from build123d import *

# Parameters (mm, degrees)
EXTRUDE_2_DEPTH      = 5
EXTRUDE_3_DEPTH      = 23.5
SKETCH_3_R           = 1.65
CUT_EXTRUDE_1_DEPTH  = 85.951456727
CUT_EXTRUDE_5_REACH  = 89.951
CUT_EXTRUDE_START    = 3
SKETCH_8_R           = 3
CUT_EXTRUDE_10_REACH = 89.951
CUT_EXTRUDE_START_2  = -3
SKETCH_12_R          = 3
SKETCH_4_W           = 20
SKETCH_4_H           = 10
CUT_EXTRUDE_2_DEPTH  = 5
SKETCH_10_W          = 16
SKETCH_10_H          = 40
CUT_EXTRUDE_11_DEPTH = 85.951456727
FILLET_1_R           = 3
CUT_EXTRUDE_6_DEPTH  = 94.465851734
SKETCH_6_R           = 2.6
CUT_EXTRUDE_3_DEPTH  = 83.421182124
CUT_EXTRUDE_4_REACH  = 89.421
CUT_EXTRUDE_START_3  = -5
SKETCH_7_R           = 4.4
FILLET_3_R           = 2
CUT_EXTRUDE_13_DEPTH = 90.709896


with BuildPart() as part:
    # 草图2 → 凸台-拉伸2 (new body)
    with BuildSketch(Plane(origin=(0, 0, 0), x_dir=(1, 0, 0), z_dir=(0, 1, 0))):
        Polygon((0, 0), (23.5, 0), (23.5, -19), (23.5, -80), (0, -80), align=None)
    extrude_2 = extrude(amount=EXTRUDE_2_DEPTH)

    # 镜向1: 凸台-拉伸2 across plane
    add(extrude_2.mirror(Plane(origin=(0, 5, 80), x_dir=(0, 0, 1), z_dir=(1, 0, 0))))

    # 草图5 → 凸台-拉伸3 (add, symmetric)
    with BuildSketch(Plane(origin=(0, 0, 0), x_dir=(0, 0, -1), z_dir=(1, 0, 0))):
        Polygon((-80, 0), (-16.263455967, -11.263455967), (-11.242997821, -6.242997821), (-9.192388155, -4.192388155), (-13.384776311, 0), align=None)
        Polygon((-13.384776311, 0), (-9.192388155, -4.192388155), (-7.14177849, -2.14177849), (-5, 0), align=None)
        Polygon((-7.14177849, -2.14177849), (-9.192388155, -4.192388155), (-8.838834765, -4.545941546), (-6.788225099, -2.495331881), align=None)
        Polygon((-9.192388155, -4.192388155), (-11.242997821, -6.242997821), (-10.88944443, -6.596551211), (-8.838834765, -4.545941546), align=None)
    extrude(amount=EXTRUDE_3_DEPTH, both=True)

    # 草图3 → 切除-拉伸1 (cut, through all)
    with BuildSketch(Plane(origin=(0, 5, 0), x_dir=(1, 0, 0), z_dir=(0, 1, 0))):
        with Locations(Location((-20, -20, 0), (0, 0, 270))):
            Circle(SKETCH_3_R)
        with Locations(Location((20, -20, 0), (0, 0, 270))):
            Circle(SKETCH_3_R)
        with Locations(Location((-20, -75, 0), (0, 0, 270))):
            Circle(SKETCH_3_R)
        with Locations(Location((20, -75, 0), (0, 0, 270))):
            Circle(SKETCH_3_R)
    extrude(amount=-CUT_EXTRUDE_1_DEPTH, mode=Mode.SUBTRACT)

    # 切除-拉伸5: up to this plane
    cut_extrude_5_end = Plane(origin=(23.5, -13.709378738, 2.422707194), z_dir=(0, 0.9847416717466503, -0.174022527063632))
    # 草图8 → 切除-拉伸5 (cut, up to the surface)
    with BuildSketch(Plane.XZ.offset(-5).offset(CUT_EXTRUDE_START), mode=Mode.PRIVATE) as cut_extrude_5_sk1:
        with Locations(Location((-20, 20, 0), (0, 0, 90))):
            Circle(SKETCH_8_R)
    cut_extrude_5_tool1 = split(extrude(cut_extrude_5_sk1.sketch, amount=CUT_EXTRUDE_5_REACH, mode=Mode.PRIVATE), bisect_by=cut_extrude_5_end, keep=Keep.BOTH, mode=Mode.PRIVATE)
    add(cut_extrude_5_tool1.solids().sort_by_distance((-20, 2, 20))[0], mode=Mode.SUBTRACT)
    # 草图8 → 切除-拉伸5 (cut, up to the surface)
    with BuildSketch(Plane.XZ.offset(-5).offset(CUT_EXTRUDE_START), mode=Mode.PRIVATE) as cut_extrude_5_sk2:
        with Locations(Location((20, 20, 0), (0, 0, 90))):
            Circle(SKETCH_8_R)
    cut_extrude_5_tool2 = split(extrude(cut_extrude_5_sk2.sketch, amount=CUT_EXTRUDE_5_REACH, mode=Mode.PRIVATE), bisect_by=cut_extrude_5_end, keep=Keep.BOTH, mode=Mode.PRIVATE)
    add(cut_extrude_5_tool2.solids().sort_by_distance((20, 2, 20))[0], mode=Mode.SUBTRACT)

    # 切除-拉伸10: up to this plane
    cut_extrude_10_end = Plane(origin=(23.5, -13.709378738, 2.422707194), z_dir=(0, 0.9847416717466503, -0.174022527063632))
    # 草图12 → 切除-拉伸10 (cut, up to the surface)
    with BuildSketch(Plane(origin=(0, 5, 0), x_dir=(1, 0, 0), z_dir=(0, 1, 0)).offset(CUT_EXTRUDE_START_2), mode=Mode.PRIVATE) as cut_extrude_10_sk1:
        with Locations(Location((-20, -75, 0), (0, 0, 270))):
            Circle(SKETCH_12_R)
    cut_extrude_10_tool1 = split(extrude(cut_extrude_10_sk1.sketch, amount=-CUT_EXTRUDE_10_REACH, mode=Mode.PRIVATE), bisect_by=cut_extrude_10_end, keep=Keep.BOTH, mode=Mode.PRIVATE)
    add(cut_extrude_10_tool1.solids().sort_by_distance((-20, 2, 75))[0], mode=Mode.SUBTRACT)
    # 草图12 → 切除-拉伸10 (cut, up to the surface)
    with BuildSketch(Plane(origin=(0, 5, 0), x_dir=(1, 0, 0), z_dir=(0, 1, 0)).offset(CUT_EXTRUDE_START_2), mode=Mode.PRIVATE) as cut_extrude_10_sk2:
        with Locations(Location((20, -75, 0), (0, 0, 270))):
            Circle(SKETCH_12_R)
    cut_extrude_10_tool2 = split(extrude(cut_extrude_10_sk2.sketch, amount=-CUT_EXTRUDE_10_REACH, mode=Mode.PRIVATE), bisect_by=cut_extrude_10_end, keep=Keep.BOTH, mode=Mode.PRIVATE)
    add(cut_extrude_10_tool2.solids().sort_by_distance((20, 2, 75))[0], mode=Mode.SUBTRACT)

    # 草图4 → 切除-拉伸2 (cut)
    with BuildSketch(Plane(origin=(0, 5, 0), x_dir=(1, 0, 0), z_dir=(0, 1, 0))):
        with Locations((0, -16)):
            Rectangle(SKETCH_4_W, SKETCH_4_H)
    extrude(amount=-CUT_EXTRUDE_2_DEPTH, mode=Mode.SUBTRACT)

    # 草图10 → 切除-拉伸11 (cut, through all)
    with BuildSketch(Plane(origin=(0, 5, 0), x_dir=(1, 0, 0), z_dir=(0, 1, 0))):
        with Locations((0, -42)):
            Rectangle(SKETCH_10_W, SKETCH_10_H)
        Polygon((-7, -72), (-15, -80), (15, -80), (7, -72), align=None)
        Polygon((23.5, -22), (15.5, -26.618802154), (15.5, -68.269538735), (23.5, -72), align=None)
        Polygon((-15.5, -26.618802154), (-23.5, -22), (-23.5, -72), (-15.5, -68.269538735), align=None)
    extrude(amount=-CUT_EXTRUDE_11_DEPTH, mode=Mode.SUBTRACT)

    # 圆角1
    fillet_1_edges = [part.edges().sort_by_distance(p)[0] for p in [
        (-23.5, -2.624849927, 22),
        (-23.5, 1.793124148, 72),
        (23.5, 1.793124148, 72),
        (23.5, -2.624849927, 22),
        (15, 2.5, 80),
        (-15, 2.5, 80),
        (-15.5, -2.216734964, 26.618802154),
        (-15.5, 1.463502525, 68.269538735),
        (15.5, 1.463502525, 68.269538735),
        (15.5, -2.216734964, 26.618802154),
        (-7, 1.793124148, 72),
        (7, 1.793124148, 72),
        (-23.5, 2.5, 80),
        (23.5, 2.5, 80),
    ]]
    fillet(fillet_1_edges, radius=FILLET_1_R)

    # 草图9 → 切除-拉伸6 (cut, through all)
    with BuildSketch(Plane(origin=(23.5, 0, 0), x_dir=(0, 0, -1), z_dir=(1, 0, 0))):
        Polygon((-5, 0), (0, 5), (0, 0), align=None)
    extrude(amount=-CUT_EXTRUDE_6_DEPTH, mode=Mode.SUBTRACT)

    # 草图6 → 切除-拉伸3 (cut, through all)
    with BuildSketch(Plane(origin=(0, 2.146446609, 2.146446609), x_dir=(1, 0, 0), z_dir=(0, -0.7071067811865459, -0.7071067811865491))):
        with Locations(Location((-13.5, 9.464466094, 0), (0, 0, 270))):
            Circle(SKETCH_6_R)
        with Locations(Location((13.5, 9.464466094, 0), (0, 0, 270))):
            Circle(SKETCH_6_R)
    extrude(amount=-CUT_EXTRUDE_3_DEPTH, mode=Mode.SUBTRACT)

    # 草图7 → 切除-拉伸4 (cut, up to next)
    with BuildSketch(Plane(origin=(0, 2.146446609, 2.146446609), x_dir=(1, 0, 0), z_dir=(0, -0.7071067811865459, -0.7071067811865491)).offset(CUT_EXTRUDE_START_3), mode=Mode.PRIVATE) as cut_extrude_4_sk1:
        with Locations((-13.5, 9.464466094)):
            Circle(SKETCH_7_R)
    cut_extrude_4_tool1 = extrude(cut_extrude_4_sk1.sketch, amount=-CUT_EXTRUDE_4_REACH, mode=Mode.PRIVATE) & part.part
    # 草图7 → 切除-拉伸4 (cut, up to next)
    with BuildSketch(Plane(origin=(0, 2.146446609, 2.146446609), x_dir=(1, 0, 0), z_dir=(0, -0.7071067811865459, -0.7071067811865491)).offset(CUT_EXTRUDE_START_3), mode=Mode.PRIVATE) as cut_extrude_4_sk2:
        with Locations((13.5, 9.464466094)):
            Circle(SKETCH_7_R)
    cut_extrude_4_tool2 = extrude(cut_extrude_4_sk2.sketch, amount=-CUT_EXTRUDE_4_REACH, mode=Mode.PRIVATE) & part.part
    add(cut_extrude_4_tool1.solids().sort_by_distance((-13.5, -1.010408, 12.374369))[0], mode=Mode.SUBTRACT)
    add(cut_extrude_4_tool2.solids().sort_by_distance((13.5, -1.010408, 12.374369))[0], mode=Mode.SUBTRACT)

    # 圆角3
    fillet_3_edges = [part.edges().sort_by_distance(p)[0] for p in [
        (0, 5, 0),
    ]]
    fillet(fillet_3_edges, radius=FILLET_3_R)

    # 草图14 → 切除-拉伸13 (cut, through all)
    with BuildSketch(Plane.ZY.offset(15.5)):
        Polygon((28.350852961, 5), (28.350852961, 0.5), (66.358327952, 3), (66.358327952, 5), align=None)
    extrude(amount=-CUT_EXTRUDE_13_DEPTH, mode=Mode.SUBTRACT)


solid = part.part
Source: CAD feature listing. Evaluate the final solid. Frame: model axes, mm. A direction names the side the tool comes from. Coordinates: 2 decimals unless noted, no trailing zeros. Loops run counter-clockwise (first coordinate to the right, second up) from the corner with the lowest first, then second, coordinate; pieces in that order, holes last. Notation, with made-up numbers: (80, -20.5) - (130, -20.5) arc R4 cw to (130, -13.5) - close; hole circle Ø2 at (15.5, -36). An arc over 180 degrees is marked (long way). One line per item, written item: value. Start each with the question number.
1. Set-up query: faces 5 (the flat face through (18.7, 2, 76.3)), 6 (the flat face through (0, 0, 62)), 7 (the cylindrical face through (23.043, 1.676, 72.319)), 8 (the cylindrical face through (-23.11, -2.89, 21.75)), 9 (the flat face through (0, 0, 16)). Return all of +Z, -Z, +X, -X, +Y, -Y with unobstructed straight access to the full face (end or side cutting, diameter ignored); none if empty.
2. Section A-A (x = 1.5). Return the cut outline in (y, z), and give its area (3 significant figures).
3. Section B-B (z = 59). Return the cut outline in (x, y), and give its area (3 significant figures).
4. Ray query, L1, parallel to X at y = 3.25, z = 75; L2, parallel to X at y = -4.75, z = 20; L3, parallel to Z at x = -20, y = -0.4. Return the intervals inside material, ascending.
5. Mould query, pull axis Z, two halves, no side actions, for faces 1 (the flat face through (0, 5, 9)), 2 (the flat face through (-12, 3, 28.351)), 3 (the flat face through (0, 0, 5)), 4 (the flat face through (-10.115, -5.553, 48.578)). Classes: pulls with the +Z half, pulls with the -Z half, needs draft (parallel to the pull), parting line crosses it, or undercut.
6. Contact query for flat-ended pins moving along their axis: P1, Ø1, axis at y = -7.5, z = 34.5, coming from the +X side; P2, Ø7.5, axis at y = -0.5, z = 48.5, coming from the -X side; P3, Ø5, axis at x = -0.5, y = 2.5, coming from the +Z side. Output: stop coordinate, or through.
7. Section C-C (z = 75). Return the cut outline in (x, y), and give its area (3 significant figures).
8. Section D-D (y = -5.5). State how many separate pieces and enclosed holes the cut face has, and give its area (3 significant figures).
Verdict:
1. face 5: -Y
1. face 6: +Y, -Y
1. face 7: +X, +Y, -Y
1. face 8: -X, +Y, -Y
1. face 9: +Y
2. outline: (-11.26, 16.26) - (-6.24, 11.24) - (-6.6, 10.89) - (-2.5, 6.79) - (-2.14, 7.14) - (1.59, 3.41) arc R2 ccw to (5, 4.83) - (5, 11) - (0, 11) - (0, 21) - (5, 21) - (5, 22) - (-10.25, 22) - close; (-3.18, 62) - (2.71, 62) - (3, 66.36) - (5, 66.36) - (5, 72) - (-1.41, 72) - close
2. area: 234 mm2
3. outline: (-15.5, -3.71) - (-8, -3.71) - (-8, 2.52) - (-15.5, 2.52) - close; (8, -3.71) - (15.5, -3.71) - (15.5, 2.52) - (8, 2.52) - close
3. area: 93.4 mm2
4. L1: x = -23.5 to -21.65, -18.35 to -10, 10 to 18.35, 21.65 to 23.5
4. L2: x = -23.5 to -23, -17 to 17, 23 to 23.5
4. L3: z = 5.4 to 17, 23 to 24.02, 70.37 to 72
5. face 1: needs draft
5. face 2: undercut
5. face 3: pulls with the -Z half
5. face 4: pulls with the +Z half
6. P1: stops at x = 15.5
6. P2: stops at x = -15.5
6. P3: stops at z = 72
7. outline: (-23.5, -0.88) - (-23, -0.88) - (-23, 2) - (-21.65, 2) - (-21.65, 5) - (-23.5, 5) - close; (-18.35, 2) - (-17, 2) - (-17, -0.88) - (-10, -0.88) - (-10, 5) - (-18.35, 5) - close; (10, -0.88) - (17, -0.88) - (17, 2) - (18.35, 2) - (18.35, 5) - (10, 5) - close; (21.65, 2) - (23, 2) - (23, -0.88) - (23.5, -0.88) - (23.5, 5) - (21.65, 5) - close
7. area: 104 mm2
8. separate pieces: 1
8. enclosed holes: 2
8. area: 946 mm2
